Input: part model. Units: mm. Frame: model coordinates. Coordinates: 2 decimals unless noted, no trailing zeros. Order: outer loops, then holes, each group sorted by start corner. A loop starts at its lowest first (then second) coordinate and runs counter-clockwise, first axis right, second up. Notation, with made-up numbers: M 78,-31 L 111,-31 A29 ccw 111,-9 Z; hole C 63.5,22.5 d8. An arc over 180 degrees is marked long. One line per item, written item: value.
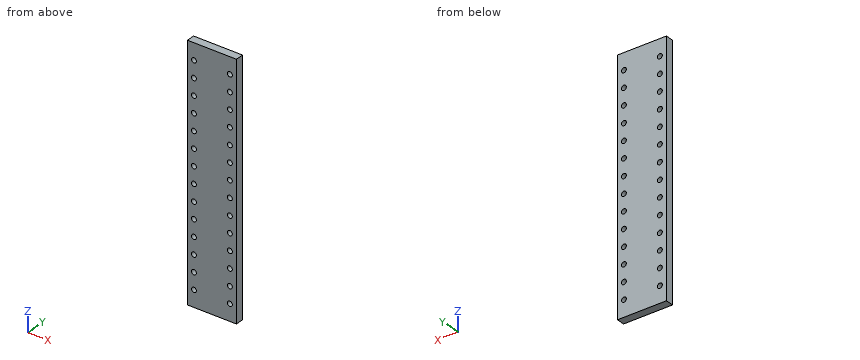
Autodesk Inventor part; units mm, degrees
ref_plane "YZ Plane" through (0, 0, 0) normal (1, 0, 0) x (0, 1, 0)
ref_plane "XZ Plane" through (0, 0, 0) normal (0, 1, 0) x (-1, 0, 0)
ref_plane "XY Plane" through (0, 0, 0) normal (0, 0, 1) x (1, 0, 0)
sketch "Sketch1" plane through (0, 0, 0) normal (0, 1, 0) x (-1, 0, 0)
  line L0 (0, 0) -> (30, 0)
  line L1 (30, 0) -> (30, -150)
  line L2 (30, -150) -> (0, -150)
  line L3 (0, -150) -> (0, 0)
  dimension "d0" = 30
  dimension "d1" = 150
extrude "Extrusion1" add sketch "Sketch1" along normal blind 5
sketch "Sketch2" plane through (0, 5, 0) normal (0, 1, 0) x (1, 0, 0)
  circle A0 centre (-26, 10) radius 1.5
  line L0 (-30, 0) -> (0, 0)
  line L1 (-30, 150) -> (-30, 0)
  circle A1 centre (-26, 20) radius 1.5
  circle A2 centre (-26, 30) radius 1.5
  circle A3 centre (-26, 40) radius 1.5
  circle A4 centre (-26, 50) radius 1.5
  circle A5 centre (-26, 60) radius 1.5
  circle A6 centre (-26, 70) radius 1.5
  circle A7 centre (-26, 80) radius 1.5
  circle A8 centre (-26, 90) radius 1.5
  circle A9 centre (-4, 10) radius 1.5
  circle A10 centre (-4, 20) radius 1.5
  circle A11 centre (-4, 30) radius 1.5
  circle A12 centre (-4, 40) radius 1.5
  circle A13 centre (-4, 50) radius 1.5
  circle A14 centre (-4, 60) radius 1.5
  circle A15 centre (-4, 70) radius 1.5
  circle A16 centre (-4, 80) radius 1.5
  circle A17 centre (-4, 90) radius 1.5
  circle A18 centre (-26, 100) radius 1.5
  circle A19 centre (-4, 100) radius 1.5
  circle A20 centre (-26, 110) radius 1.5
  circle A21 centre (-4, 110) radius 1.5
  circle A22 centre (-26, 120) radius 1.5
  circle A23 centre (-4, 120) radius 1.5
  circle A24 centre (-26, 130) radius 1.5
  circle A25 centre (-4, 130) radius 1.5
  circle A26 centre (-26, 140) radius 1.5
  circle A27 centre (-4, 140) radius 1.5
  dimension "d4" = 3
  dimension "d5" = 10
  dimension "d6" = 4
  dimension "d9" = 10
  dimension "d12" = 22
extrude "Extrusion2" cut sketch "Sketch2" against normal blind 5
properties part number "board" material "Wood (Cherry)"
(1) Cut plane A-A on y = 3. Give the number of separate pieces and of enclosed holes in the cut face, plus the area to 3 significant figures.
Data:
separate pieces: 1
enclosed holes: 28
area: 4,300 mm2
(2) Cut plane B-B on z = -10. Output: boundary loops of the cut face in (x, y), plus the area to 3 significant figures.
Data:
outline: M -30,0 L -27.5,0 L -27.5,5 L -30,5 Z; M -24.5,0 L -5.5,0 L -5.5,5 L -24.5,5 Z; M -2.5,0 L 0,0 L 0,5 L -2.5,5 Z
area: 120 mm2
(3) Ray query, line 1 (X direction, y = 2.8, z = -10); line 2 (X direction, y = 0.75, z = -110.5). Return the intervals inside material, ascending. Write a range as from..to.
Data:
line 1: x = -30..-27.5, -24.5..-5.5, -2.5..0
line 2: x = -30..-27.41, -24.59..-5.41, -2.59..0
